Verification items for the finished model (mm, model axes). A direction names the side the tool comes from. Coordinates: 2 decimals unless noted, no trailing zeros. Write each loop counter-clockwise with the first axis right and the second up, starting at its lowest first coordinate (ties: lowest second). Pieces come first, ordered by that corner, then holes. Notation, with made-up numbers: (31, -35.5) -> (73, -35.5) arc R6 cw to (73, -27.5) -> close; hole circle Ø11 at (-11.5, -27.5). An arc over 180 degrees is marked (long way). Answer in a Markdown table with one row per item.
```python
from build123d import *

# Parameters (mm, degrees)
SKETCH1_W                       = 461.66024
SKETCH1_H                       = 381
BOSS_EXTRUDE1_DEPTH             = 0.9144
EDGE_FLANGE1_STRIP_W            = 5.4864
EDGE_FLANGE1_STRIP_H            = 0.9144
EDGE_FLANGE1_STRIP_CUT_DEPTH    = 381
EDGE_FLANGE1_DEPTH              = 381
EDGE_FLANGE2_STRIP_W            = 5.4864
EDGE_FLANGE2_STRIP_H            = 0.9144
EDGE_FLANGE2_STRIP_CUT_DEPTH    = 381
EDGE_FLANGE2_DEPTH              = 381
F_0_257_DIAMETER_HOLE1_D        = 6.5278
F_0_257_DIAMETER_HOLE2_D        = 6.5278
SKETCH17_R                      = 57.15
CUT_EXTRUDE1_DEPTH              = 301.990559914
F_5_0_5_DIAMETER_HOLE1_D        = 5
F_1_4_0_25_DIAMETER_SLOT1_DEPTH = 0.9144
LPATTERN1_COUNT                 = 8
LPATTERN1_PITCH                 = 25.4
LPATTERN1_COL_COUNT             = 8
LPATTERN1_COL_PITCH             = 25.4


# Read off the part's stored shape, not the designer's step: 1/4 (0.25) Diameter Slot1
# Sheet-metal steps are written as plain solids
with BuildPart() as part:
    # Sketch1 → Boss-Extrude1 (new body)
    with BuildSketch(Plane.XY):
        Rectangle(SKETCH1_W, SKETCH1_H)
    extrude(amount=BOSS_EXTRUDE1_DEPTH)

    # Edge-Flange1 strip (across the edge) → Edge-Flange1 strip cut (cut)
    with BuildSketch(Plane(origin=(230.83012, -190.5, 0.9144), x_dir=(-1, 0, 0), z_dir=(0, 1, 0))):
        with Locations((-1.8288, -0.4572)):
            Rectangle(EDGE_FLANGE1_STRIP_W, EDGE_FLANGE1_STRIP_H)
    extrude(amount=EDGE_FLANGE1_STRIP_CUT_DEPTH, mode=Mode.SUBTRACT)

    # Edge-Flange1 section (across the edge) → Edge-Flange1 (add)
    with BuildSketch(Plane(origin=(230.83012, -190.5, 0.9144), x_dir=(-1, 0, 0), z_dir=(0, 1, 0))):
        with BuildLine():
            Line((-0.9144, 0.9144), (-0.9144, 24.4856))
            Line((-0.9144, 24.4856), (0, 24.4856))
            Line((0, 24.4856), (0, 0.9144))
            ThreePointArc((0, 0.9144), (0.267821559, 0.267821559), (0.9144, 0))
            Line((0.9144, 0), (0.9144, -0.9144))
            ThreePointArc((0.9144, -0.9144), (-0.378756881, -0.378756881), (-0.9144, 0.9144))
        make_face()
    extrude(amount=EDGE_FLANGE1_DEPTH)

    # Edge-Flange2 strip (across the edge) → Edge-Flange2 strip cut (cut)
    with BuildSketch(Plane(origin=(-230.83012, 190.5, 0.9144), x_dir=(1, 0, 0), z_dir=(0, -1, 0))):
        with Locations((-1.8288, -0.4572)):
            Rectangle(EDGE_FLANGE2_STRIP_W, EDGE_FLANGE2_STRIP_H)
    extrude(amount=EDGE_FLANGE2_STRIP_CUT_DEPTH, mode=Mode.SUBTRACT)

    # Edge-Flange2 section (across the edge) → Edge-Flange2 (add)
    with BuildSketch(Plane(origin=(-230.83012, 190.5, 0.9144), x_dir=(1, 0, 0), z_dir=(0, -1, 0))):
        with BuildLine():
            Line((-0.9144, 0.9144), (-0.9144, 24.4856))
            Line((-0.9144, 24.4856), (0, 24.4856))
            Line((0, 24.4856), (0, 0.9144))
            ThreePointArc((0, 0.9144), (0.267821559, 0.267821559), (0.9144, 0))
            Line((0.9144, 0), (0.9144, -0.9144))
            ThreePointArc((0.9144, -0.9144), (-0.378756881, -0.378756881), (-0.9144, 0.9144))
        make_face()
    extrude(amount=EDGE_FLANGE2_DEPTH)

    # F (0.257) Diameter Hole1 (through all)
    with Locations(Plane.ZY.offset(231.74452)):
        with Locations((13.6144, 76.2), (13.6144, 0), (13.6144, -76.2), (13.6144, -152.4), (13.6144, 152.4)):
            Hole(F_0_257_DIAMETER_HOLE1_D / 2)

    # F (0.257) Diameter Hole2 (through all)
    with Locations(Plane(origin=(0, 0, 0), x_dir=(-1, 0, 0), z_dir=(0, 0, -1))):
        with Locations((217.21572, 152.4), (-217.21572, 152.4), (-217.21572, 76.2), (-217.21572, 0), (-217.21572, -76.2), (-217.21572, -152.4), (217.21572, -152.4), (217.21572, -76.2), (217.21572, 0), (217.21572, 76.2)):
            Hole(F_0_257_DIAMETER_HOLE2_D / 2)

    # Sketch17 → Cut-Extrude1 (cut, through all)
    with BuildSketch(Plane.XY.offset(0.9144)):
        with Locations((0, 63.5)):
            Circle(SKETCH17_R)
    extrude(amount=-CUT_EXTRUDE1_DEPTH, mode=Mode.SUBTRACT)

    # Ø5.0 (5) Diameter Hole1 (through all)
    with Locations(Plane.XY.offset(0.9144)):
        with Locations((0, 63.5), (52.5, 116), (-52.5, 11), (-52.5, 116), (52.5, 11)):
            Hole(F_5_0_5_DIAMETER_HOLE1_D / 2)

    # 1/4 (0.25) Diameter Slot1 outline → 1/4 (0.25) Diameter Slot1 (cut)
    with BuildSketch(Plane.XY):
        with BuildLine():
            Line((3.175, -136.525), (3.175, -92.075))
            ThreePointArc((3.175, -92.075), (0, -88.9), (-3.175, -92.075))
            Line((-3.175, -92.075), (-3.175, -136.525))
            ThreePointArc((-3.175, -136.525), (0, -139.7), (3.175, -136.525))
        make_face()
    f_1_4_0_25_diameter_slot1 = extrude(amount=F_1_4_0_25_DIAMETER_SLOT1_DEPTH, mode=Mode.SUBTRACT)

    # LPattern1: 1/4 (0.25) Diameter Slot1 ×8
    with Locations(*[(-i * LPATTERN1_PITCH, 0, 0) for i in range(1, LPATTERN1_COUNT)]):
        add(f_1_4_0_25_diameter_slot1, mode=Mode.SUBTRACT)

    # LPattern1 col: 1/4 (0.25) Diameter Slot1 ×8
    with Locations(*[(i * LPATTERN1_COL_PITCH, 0, 0) for i in range(1, LPATTERN1_COL_COUNT)]):
        add(f_1_4_0_25_diameter_slot1, mode=Mode.SUBTRACT)


solid = part.part
```
1. Tool access check on faces 1 (the cylindrical face through (-12.39, 7.71, 0.46)), 2 (the flat face through (-230.83, 3, 16)). Record the directions out of +Z, -Z, +X, -X, +Y, -Y that give a thin tool (end or side, any length) a straight path to the whole face; none if there is none.
Geometry says:
| item | result |
|---|---|
| face 1 | +Z, -Z |
| face 2 | +Z, +Y, -Y |
2. Mould release check, pull along X, two halves, no side actions. Record for faces 3 (the flat face through (230.83, -3, 16)), 4 (the flat face through (1.1, -190.5, 0.5)), 5 (the flat face through (-231.745, 3, 11)), 6 (the flat face through (-3, 3, 0.914)): released by +X, released by -X, zero draft, split by the parting line, or undercut.
Geometry says:
| item | result |
|---|---|
| face 3 | undercut |
| face 4 | zero draft |
| face 5 | released by -X |
| face 6 | undercut |
3. Section check C-C, the plane y = -118. State how many separate pieces and enclosed holes the cut face has, plus the area to 3 significant figures.
Geometry says:
| item | result |
|---|---|
| separate pieces | 16 |
| enclosed holes | 0 |
| area | 380 mm^2 |
4. Section check B-B, the plane y = 45.5. Record the boundary of the cut face in (x, z), plus the area to 3 significant figures.
Geometry says:
| item | result |
|---|---|
| outline | (-231.74, 1.83) arc R1.83 ccw to (-229.92, 0) -> (-54.24, 0) -> (-54.24, 0.91) -> (-229.92, 0.91) arc R0.91 cw to (-230.83, 1.83) -> (-230.83, 25.4) -> (-231.74, 25.4) -> close; (54.24, 0) -> (229.92, 0) arc R1.83 ccw to (231.74, 1.83) -> (231.74, 25.4) -> (230.83, 25.4) -> (230.83, 1.83) arc R0.91 cw to (229.92, 0.91) -> (54.24, 0.91) -> close |
| area | 368 mm^2 |
5. Thickness scan on line 1 (X direction, y = -152.4, z = 0.2); line 2 (X direction, y = 56, z = 17); line 3 (X direction, y = -152.4, z = 0.4). Record the ranges inside material, lowest first. Write a range as from..to.
Geometry says:
| item | result |
|---|---|
| line 1 | -230.75..-220.48, -213.95..213.95, 220.48..230.75 |
| line 2 | -231.74..-230.83, 230.83..231.74 |
| line 3 | -231.06..-220.48, -213.95..213.95, 220.48..231.06 |
6. Section check A-A, the plane y = -166.5. Record the boundary of the cut face in (x, z), plus the area to 3 significant figures.
Geometry says:
| item | result |
|---|---|
| outline | (-231.74, 1.83) arc R1.83 ccw to (-229.92, 0) -> (229.92, 0) arc R1.83 ccw to (231.74, 1.83) -> (231.74, 25.4) -> (230.83, 25.4) -> (230.83, 1.83) arc R0.91 cw to (229.92, 0.91) -> (-229.92, 0.91) arc R0.91 cw to (-230.83, 1.83) -> (-230.83, 25.4) -> (-231.74, 25.4) -> close |
| area | 468 mm^2 |
7. Section check D-D, the plane x = 165.5. Record the boundary of the cut face in (y, z).
Geometry says:
| item | result |
|---|---|
| outline | (-190.5, 0) -> (190.5, 0) -> (190.5, 0.91) -> (-190.5, 0.91) -> close |
8. Depth check by flat-ended pin: P1, Ø0.7, axis at y = -114, z = 0.5, coming from the +X side; P2, Ø0.7, axis at y = -119.5, z = 0.5, coming from the -X side; P3, Ø0.5, axis at y = -104.5, z = 0.5, coming from the +X side. Enter the tip coordinate at first touch or a pass-through.
Geometry says:
| item | result |
|---|---|
| P1 | x = 231.46 |
| P2 | x = -231.46 |
| P3 | x = 231.39 |
